Could you check a few things on this drawing? It's one solid part, dimensions in mm from its lowest x, y, z. Round coordinates to 2 decimals unless told otherwise and drop trailing zeros. Write each loop counter-clockwise with the first axis right and the second up, starting at its lowest first coordinate (ties: lowest second). Pieces come first, ordered by that corner, then holes. Notation, with made-up numbers: (51.25, 61) -> (56.25, 61) arc R6 cw to (56.25, 71) -> close; hole circle Ø8 at (39.25, 32). An arc over 180 degrees is marked (long way). Answer in a Markdown table with one row per item.
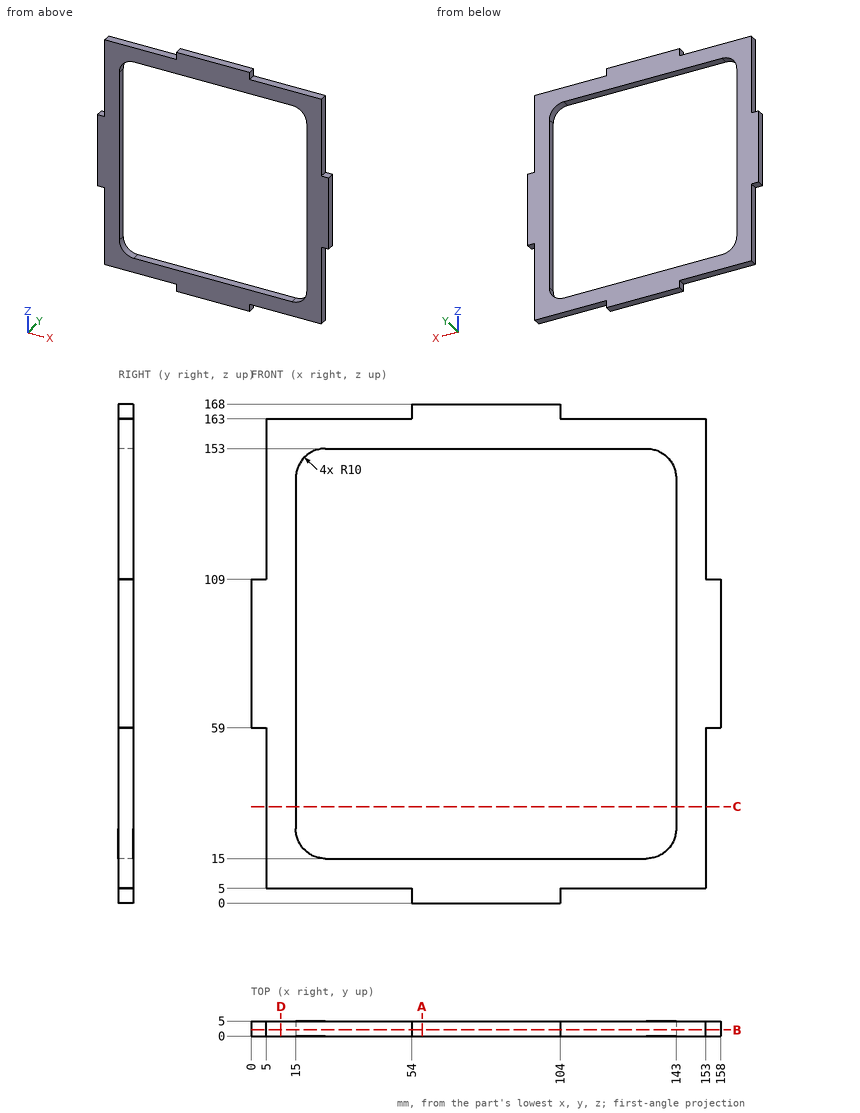
1) I want a section at D-D, the plane x = 10. List the corners of the cut face in (y, z) for me.
Response:
| item | result |
|---|---|
| outline | (0, 5) -> (5, 5) -> (5, 163) -> (0, 163) -> close |
2) I need wall thicknesses on line 1 (X direction, y = 3.3, z = 132); line 2 (Z direction, x = 50.5, y = 1.1); line 3 (X direction, y = 2.1, z = 101). Which ranges of each line are inside material? Lowest first, please. Write a range as [from, to].
Response:
| item | result |
|---|---|
| line 1 | x = [5, 15], [143, 153] |
| line 2 | z = [5, 15], [153, 163] |
| line 3 | x = [0, 15], [143, 158] |
3) For pin 1 (1.5 mm diameter, centred on x = 155, y = 2, fed in from +Z); pin 2 (1.5 mm diameter, centred on x = 22.5, y = 3.5, fed in from -Z); pin 3 (1 mm diameter, centred on x = 46.5, y = 4, fed in from +Z), each with a flat end and sliding along its axis, tell me the tip position at first contact or that it passes through.
Response:
| item | result |
|---|---|
| pin 1 | stops at z = 109 |
| pin 2 | stops at z = 5 |
| pin 3 | stops at z = 163 |
4) I want a section at B-B, the plane y = 2.1. List the corners of the cut face in (x, z) for me.
Response:
| item | result |
|---|---|
| outline | (0, 59) -> (5, 59) -> (5, 5) -> (54, 5) -> (54, 0) -> (104, 0) -> (104, 5) -> (153, 5) -> (153, 59) -> (158, 59) -> (158, 109) -> (153, 109) -> (153, 163) -> (104, 163) -> (104, 168) -> (54, 168) -> (54, 163) -> (5, 163) -> (5, 109) -> (0, 109) -> close; hole (15, 25) arc R10 ccw to (25, 15) -> (133, 15) arc R10 ccw to (143, 25) -> (143, 143) arc R10 ccw to (133, 153) -> (25, 153) arc R10 ccw to (15, 143) -> close |
5) I want a section at A-A, the plane x = 57.5. List the corners of the cut face in (y, z) for me, and give its area (3 significant figures).
Response:
| item | result |
|---|---|
| outline | (0, 0) -> (5, 0) -> (5, 15) -> (0, 15) -> close; (0, 153) -> (5, 153) -> (5, 168) -> (0, 168) -> close |
| area | 150 mm^2 |
6) I want a section at C-C, the plane z = 32.5. List the corners of the cut face in (x, y) for me.
Response:
| item | result |
|---|---|
| outline | (5, 0) -> (15, 0) -> (15, 5) -> (5, 5) -> close; (143, 0) -> (153, 0) -> (153, 5) -> (143, 5) -> close |
